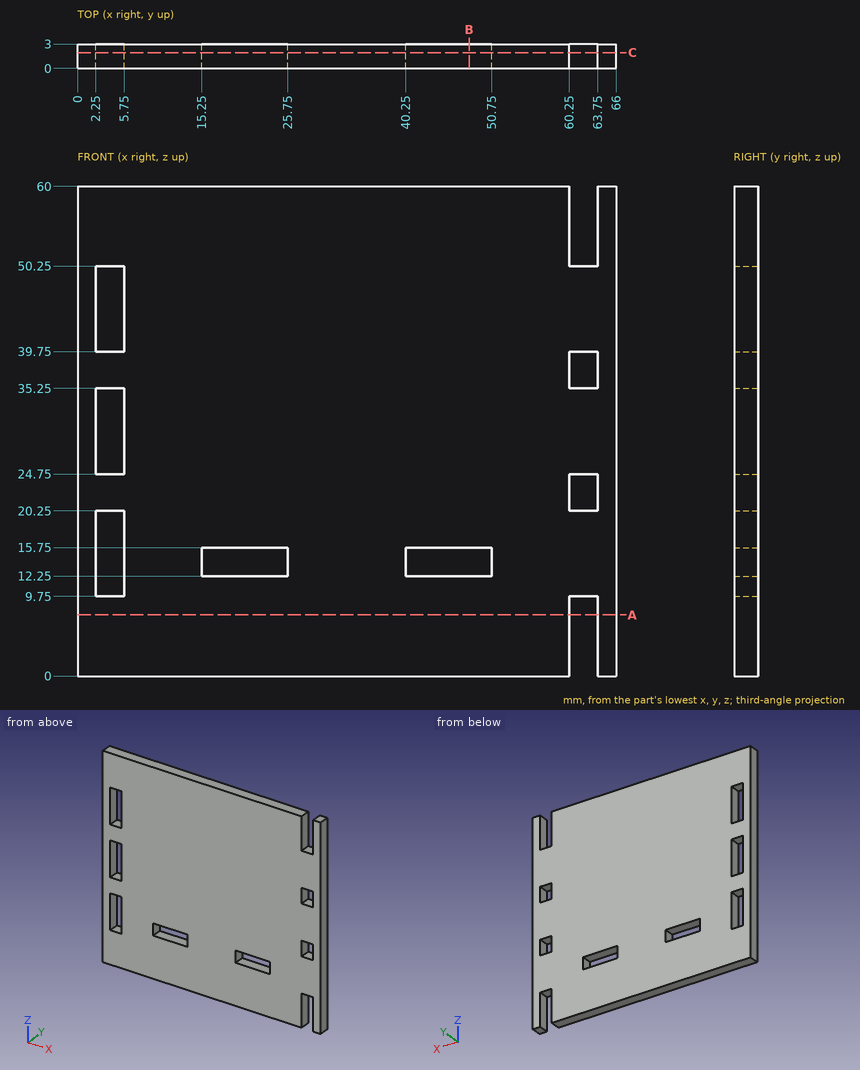
Geometry: see drawing. Coordinates: mm, zero at the bounding-box minimum. Give positions to 0.01 mm unless a question says otherwise; leave off trailing zeros. Order: outer loops, then holes, each group sorted by start corner. A loop starts at its lowest first (then second) coordinate and runs counter-clockwise, first axis right, second up. Notation, with made-up numbers: (6, 70) -> (26, 70) arc R20 cw to (26, 96) -> close; hole circle Ø5 at (89.5, 77). An arc over 180 degrees is marked (long way). Write each question's results on one line, items separated by ' | '.
1) Line query: line 1 along X through (y, z) = (0.35, 13); line 2 along Z through (x, y) = (23, 0.95); line 3 along X through (y, z) = (0.6, 35). Output: solid intervals per line, ascending.
Geometry says:
line 1: x = 0 to 2.25, 5.75 to 15.25, 25.75 to 40.25, 50.75 to 66 | line 2: z = 0 to 12.25, 15.75 to 60 | line 3: x = 0 to 2.25, 5.75 to 66
2) Cut plane B-B (x = 48). Output: boundary loops of the cut face in (y, z).
Geometry says:
outline: (0, 0) -> (3, 0) -> (3, 12.25) -> (0, 12.25) -> close; (0, 15.75) -> (3, 15.75) -> (3, 60) -> (0, 60) -> close
3) Cut plane A-A (z = 7.5). Output: boundary loops of the cut face in (x, y).
Geometry says:
outline: (0, 0) -> (60.25, 0) -> (60.25, 3) -> (0, 3) -> close; (63.75, 0) -> (66, 0) -> (66, 3) -> (63.75, 3) -> close
4) Cut plane C-C (y = 1.95). Give the number of separate pieces and of enclosed holes in the cut face, and give its area (3 significant figures).
Geometry says:
separate pieces: 1 | enclosed holes: 7 | area: 3,680 mm²
